Part model, mm, in its own coordinate system. A direction names the side the tool comes from. Round coordinates to 2 decimals unless told otherwise and drop trailing zeros. Loops run counter-clockwise (first coordinate to the right, second up) from the corner with the lowest first, then second, coordinate; pieces in that order, holes last. Notation, with made-up numbers: (-33.5, 12.5) -> (-16.5, 12.5) arc R29 ccw to (-16.5, 41.5) -> close; hole circle Ø5 at (5.5, 9.25). An arc over 180 degrees is marked (long way). Answer as a JSON object with one key per item and string values. Group by question number.
from build123d import *

# Parameters (mm, degrees)
F1_DEPTH  = 250
F2_W      = 87.5
F2_H      = 12
F3_DEPTH  = 20
F5_D      = 7
F5_DEPTH  = 40
F5_TIP    = 2.1030121666
F7_DEPTH  = 17
F8_DEPTH  = 17
F9_W      = 16.9
F9_H      = 250
F10_DEPTH = 10
F11_W     = 16.9
F11_H     = 250
F12_DEPTH = 10
F14_DEPTH = 25
F15_R     = 5
F18_W     = 250
F18_H     = 10
F19_DEPTH = 0.1
F20_W     = 250
F20_H     = 10
F21_DEPTH = 0.1
F22_W     = 143.5878481716
F22_H     = 63.6908710003
F23_DEPTH = 259


with BuildPart() as f1:
    # F0 (on Front) → F1 (new body)
    with BuildSketch(Plane.XZ):
        Polygon((-45.825098525, 2), (-45.825098525, 0), (41.674901475, 0), (41.674901475, 2), (21.674901475, 2), (21.674901475, 12), (-25.825098525, 12), (-25.825098525, 2), align=None)
    extrude(amount=F1_DEPTH)

    # F2 (on face) → F3 (join)
    with BuildSketch(Plane(origin=(0, 0, 0), x_dir=(-1, 0, 0), z_dir=(0, 1, 0))):
        with Locations((2.075098525, 6)):
            Rectangle(F2_W, F2_H)
    extrude(amount=F3_DEPTH)

    # F5
    with Locations(Plane.XY.offset(2)):
        with Locations((-35.825098525, -51), (31.674901475, -199), (31.674901475, -51), (-35.825098525, -199)):
            Hole(F5_D / 2, depth=F5_DEPTH)
            with Locations((0, 0, -(F5_DEPTH + F5_TIP / 2))):  # 118° drill point
                Cone(0, F5_D / 2, F5_TIP, mode=Mode.SUBTRACT)

    # F7 (add): a face of the model
    f7_faces = [f1.faces().sort_by_distance(p)[0] for p in [
        (-45.825098525, -125, 1.7297334649),
    ]]
    extrude(f7_faces, amount=F7_DEPTH)

    # F6 (on face) → F8 (join)
    with BuildSketch(Plane.YZ.offset(41.674901475)):
        Polygon((0, 2), (-250, 2), (-250, 0), (20, 0), (20, 12), (0, 12), align=None)
    extrude(amount=F8_DEPTH)

    # F9 (on face) → F10 (join)
    with BuildSketch(Plane.XY.offset(2)):
        with Locations((50.224901475, -125)):
            Rectangle(F9_W, F9_H)
    extrude(amount=F10_DEPTH)

    # F11 (on face) → F12 (join)
    with BuildSketch(Plane.XY.offset(2)):
        with Locations((-54.375098525, -125)):
            Rectangle(F11_W, F11_H)
    extrude(amount=F12_DEPTH)

    # F13 (on face) → F14 (cut)
    with BuildSketch(Plane.XY.offset(12)):
        with BuildLine():
            ThreePointArc((-62.825098525, 0), (-37.10740093, 13.9610044228), (-8.4745501026, 20))
            Line((-8.4745501026, 20), (-62.825098525, 20))
            Line((-62.825098525, 20), (-62.825098525, 0))
        make_face()
        with BuildLine():
            ThreePointArc((4.3243530527, 20), (32.95720388, 13.9610044228), (58.674901475, 0))
            Line((58.674901475, 0), (58.674901475, 20))
            Line((58.674901475, 20), (4.3243530527, 20))
        make_face()
    extrude(amount=-F14_DEPTH, mode=Mode.SUBTRACT)

    # F15
    f15_edges = [f1.edges().sort_by_distance(p)[0] for p in [
        (-37.107401, 13.961004, 12),
        (-2.075099, 20, 12),
        (32.957204, 13.961004, 12),
    ]]
    fillet(f15_edges, radius=F15_R)

    # F18 (on face) → F19 (cut)
    with BuildSketch(Plane.YZ.offset(21.674901475)):
        with Locations((-125, 7)):
            Rectangle(F18_W, F18_H)
    extrude(amount=-F19_DEPTH, mode=Mode.SUBTRACT)

    # F20 (on face) → F21 (cut)
    with BuildSketch(Plane(origin=(-25.825098525, 0, 0), x_dir=(0, -1, 0), z_dir=(-1, 0, 0))):
        with Locations((125, 7)):
            Rectangle(F20_W, F20_H)
    extrude(amount=-F21_DEPTH, mode=Mode.SUBTRACT)

    # F22 (on offset) → F23 (cut)
    with BuildSketch(Plane(origin=(-112.825098525, 0, 0), x_dir=(0, -1, 0), z_dir=(-1, 0, 0))):
        with Locations((44.3292455748, 5.149319768)):
            Rectangle(F22_W, F22_H)
    extrude(amount=-F23_DEPTH, mode=Mode.SUBTRACT)


solid = f1.part
Item 1: Band-saw the part on B-B, the plane z = 10.5. List the corners of the cut face in (x, y).
Item 2: Two-plate mould, pull along X, no slides. Class faces 1 (the face through (-2, -182, 12)), 2 (the face through (-36, -182, 2)), 3 (the face through (-62.825, -184, 6)), 4 (the face through (58.675, -184, 6)): pulls with the +X half, pulls with the -X half, needs draft (parallel to the pull), parting line crosses it, or undercut.
Item 3: Which spindle directions (+Z, -Z, +X, -X, +Y, -Y) get a long thin tool onto all of the face, cutting with end or side? Do faces 5 (the face through (-3, -250, 5)), 6 (the face through (-45.925, -184, 7)). Say none if no direction does.
Item 4: Drop flat-ended pins along their axis: pin 1 Ø3 at (x, y) = (35, -141) entering from +Z; pin 2 Ø6.5 at (x, y) = (31.67, -199) entering from -Z (3 decimals). Give the stop position or say it passes through.
Item 5: Drill centre lines: line 1 (X direction, y = -175, z = 11.5); line 2 (X direction, y = -199, z = 0.5); line 3 (Z direction, x = 36, y = -240). Where is each one in solid material? Low to high.
Item 6: Band-saw the part on D-D, the plane x = 33. List the corners of the cut face in (y, z), plus the area to 3 significant figures.
Item 7: Band-saw the part on C-C, the plane y = -182.5. List the corners of the cut face in (x, z), plus the area to 3 significant figures.
Item 8: Band-saw the part on A-A, the plane y = -199. List the corners of the cut face in (x, z).
Entries:
{
 "1": {"outline": "(-62.83, -250) -> (-45.93, -250) -> (-45.93, -116.12) -> (-62.83, -116.12) -> close; (-25.73, -250) -> (21.57, -250) -> (21.57, -116.12) -> (-25.73, -116.12) -> close; (41.77, -250) -> (58.67, -250) -> (58.67, -116.12) -> (41.77, -116.12) -> close"},
 "2": {"face 1": "needs draft", "face 2": "undercut", "face 3": "pulls with the -X half", "face 4": "pulls with the +X half"},
 "3": {"face 5": "+Z, -Z, +X, -X, -Y", "face 6": "+Z, +Y, -Y"},
 "4": {"pin 1": "z = 2", "pin 2": "through"},
 "5": {"line 1": "-62.83 to -45.93, -25.73 to 21.57, 41.77 to 58.67", "line 2": "-62.83 to -39.33, -32.33 to 28.17, 35.17 to 58.67", "line 3": "0 to 2"},
 "6": {"outline": "(-250, 0) -> (-202.24, 0) -> (-202.24, 2) -> (-250, 2) -> close; (-195.76, 0) -> (-116.12, 0) -> (-116.12, 2) -> (-195.76, 2) -> close", "area": "255 mm²"},
 "7": {"outline": "(-62.83, 0) -> (58.67, 0) -> (58.67, 12) -> (41.77, 12) -> (41.77, 2) -> (21.57, 2) -> (21.57, 12) -> (-25.73, 12) -> (-25.73, 2) -> (-45.93, 2) -> (-45.93, 12) -> (-62.83, 12) -> close", "area": "1,050 mm²"},
 "8": {"outline": "(-62.83, 0) -> (-39.33, 0) -> (-39.33, 2) -> (-45.93, 2) -> (-45.93, 12) -> (-62.83, 12) -> close; (-32.33, 0) -> (28.17, 0) -> (28.17, 2) -> (21.57, 2) -> (21.57, 12) -> (-25.73, 12) -> (-25.73, 2) -> (-32.33, 2) -> close; (35.17, 0) -> (58.67, 0) -> (58.67, 12) -> (41.77, 12) -> (41.77, 2) -> (35.17, 2) -> close"}
}
